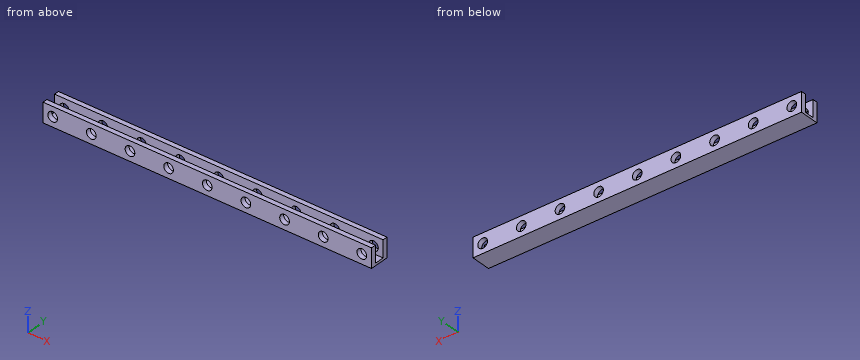
from build123d import *

# Parameters (mm, degrees)
SKETCH1_W           = 136
SKETCH1_H           = 8
BOSS_EXTRUDE1_DEPTH = 8
SKETCH2_W           = 7
SKETCH2_H           = 4
CUT_EXTRUDE1_DEPTH  = 142
SKETCH3_R           = 2
CUT_EXTRUDE2_DEPTH  = 142


with BuildPart() as part:
    # Sketch1 → Boss-Extrude1 (new body)
    with BuildSketch(Plane(origin=(0, 0, 0), x_dir=(1, 0, 0), z_dir=(0, 1, 0))):
        with Locations((-1.696732132, 28.439939714)):
            Rectangle(SKETCH1_W, SKETCH1_H)
    extrude(amount=BOSS_EXTRUDE1_DEPTH)

    # Sketch2 → Cut-Extrude1 (cut)
    with BuildSketch(Plane.ZY.offset(69.696732132)):
        with Locations((-27.939939714, 4)):
            Rectangle(SKETCH2_W, SKETCH2_H)
    extrude(amount=-CUT_EXTRUDE1_DEPTH, mode=Mode.SUBTRACT)

    # Sketch3 → Cut-Extrude2 (cut)
    with BuildSketch(Plane(origin=(0, 8, 0), x_dir=(1, 0, 0), z_dir=(0, 1, 0))):
        with Locations(Location((-65.696732132, 28.439939714, 0), (0, 0, 270))):
            Circle(SKETCH3_R)
        with Locations(Location((-49.696732132, 28.439939714, 0), (0, 0, 270))):
            Circle(SKETCH3_R)
        with Locations(Location((-33.696732132, 28.439939714, 0), (0, 0, 270))):
            Circle(SKETCH3_R)
        with Locations(Location((-17.696732132, 28.439939714, 0), (0, 0, 270))):
            Circle(SKETCH3_R)
        with Locations(Location((-1.696732132, 28.439939714, 0), (0, 0, 270))):
            Circle(SKETCH3_R)
        with Locations(Location((14.303267868, 28.439939714, 0), (0, 0, 270))):
            Circle(SKETCH3_R)
        with Locations(Location((30.303267868, 28.439939714, 0), (0, 0, 270))):
            Circle(SKETCH3_R)
        with Locations(Location((46.303267868, 28.439939714, 0), (0, 0, 270))):
            Circle(SKETCH3_R)
        with Locations(Location((62.303267868, 28.439939714, 0), (0, 0, 270))):
            Circle(SKETCH3_R)
    extrude(amount=-CUT_EXTRUDE2_DEPTH, mode=Mode.SUBTRACT)


solid = part.part
Build history of the part. All positions in model axes, mm. Round coordinates to 2 decimals unless told otherwise and drop trailing zeros. Loops run counter-clockwise (first coordinate to the right, second up) from the corner with the lowest first, then second, coordinate; pieces in that order, holes last. Notation, with made-up numbers: (30.5, 24) -> (35.5, 24) arc R17 ccw to (35.5, 36) -> close; hole circle Ø3 at (10, -33). An arc over 180 degrees is marked (long way). Use CSV: the item, a comma, the result in double quotes. Start each with the question number.
Q1. Saw through at A-A on x = -59. Give the cut face in (y, z).
Q2. Saw through at C-C on y = 3.25. Give the cut face in (x, z), and give its area (3 significant figures).
Q3. Drill centre lines: L1, parallel to Y at x = 37.5, z = -31; L2, parallel to Z at x = 58.5, y = 3.5. Where is each one in solid material? Low to high.
Q4. Flat gauge pin, fed straight in: pin 1 Ø3 at (x, z) = (14.3, -28.44) entering from -Y. Where does the tip first touch, or does it go through?
Q5. Saw through at B-B on z = -27.75. Count the separate pieces of the cut face and the enclosed holes in it, and give its area (3 significant figures).
Solutions:
1,outline,"(0, -32.44) -> (8, -32.44) -> (8, -24.44) -> (6, -24.44) -> (6, -31.44) -> (2, -31.44) -> (2, -24.44) -> (0, -24.44) -> close"
2,outline,"(-69.7, -32.44) -> (66.3, -32.44) -> (66.3, -31.44) -> (-69.7, -31.44) -> close"
2,area,"136 mm^2"
3,L1,"y = 0 to 2, 6 to 8"
3,L2,"z = -32.44 to -31.44"
4,pin 1,"passes through"
5,separate pieces,"20"
5,enclosed holes,"0"
5,area,"409 mm^2"
